Work out the finished part from the listing and answer in its coordinate system (mm). Give positions to 0.01 mm unless a question says otherwise; leave off trailing zeros. Write each loop counter-clockwise with the first axis right and the second up, starting at its lowest first coordinate (ties: lowest second). Pieces come first, ordered by that corner, then holes. Notation, with made-up numbers: (26.5, -9) - (52.5, -9) arc R25 ccw to (52.5, 12) - close; hole circle Ø4 at (87, 17). An arc over 180 degrees is marked (long way). Write item = value, one per line.
from build123d import *

# Parameters (mm, degrees)
F0_R     = 3.05
F0_R_2   = 2.5
F1_DEPTH = 5
F2_SIZE  = 3.5


with BuildPart() as f1:
    # F0 (on Top) → F1 (new body)
    with BuildSketch(Plane.XY):
        with BuildLine():
            Line((0, 225), (0, 0))
            Line((0, 0), (72.5, 0))
            ThreePointArc((72.5, 0), (86.642136, -5.857864), (92.5, -20))
            Line((92.5, -20), (92.5, -50))
            ThreePointArc((92.5, -50), (98.357864, -64.142136), (112.5, -70))
            Line((112.5, -70), (152.5, -70))
            ThreePointArc((152.5, -70), (166.642136, -64.142136), (172.5, -50))
            Line((172.5, -50), (172.5, -20))
            ThreePointArc((172.5, -20), (178.357864, -5.857864), (192.5, 0))
            Line((192.5, 0), (265, 0))
            Line((265, 0), (265, 225))
            Line((265, 225), (0, 225))
        make_face()
        with Locations((112.5, -50)):
            Circle(F0_R, mode=Mode.SUBTRACT)
        with Locations((112.5, -10)):
            Circle(F0_R, mode=Mode.SUBTRACT)
        with Locations((11, 35)):
            Circle(F0_R_2, mode=Mode.SUBTRACT)
        with Locations((11, 54.5)):
            Circle(F0_R_2, mode=Mode.SUBTRACT)
        with Locations((152.5, -50)):
            Circle(F0_R, mode=Mode.SUBTRACT)
        with Locations((152.5, -10)):
            Circle(F0_R, mode=Mode.SUBTRACT)
        with Locations((254, 35)):
            Circle(F0_R_2, mode=Mode.SUBTRACT)
        with Locations((254, 54.5)):
            Circle(F0_R_2, mode=Mode.SUBTRACT)
        with Locations((11, 170.5)):
            Circle(F0_R_2, mode=Mode.SUBTRACT)
        with Locations((11, 190)):
            Circle(F0_R_2, mode=Mode.SUBTRACT)
        with Locations((254, 170.5)):
            Circle(F0_R_2, mode=Mode.SUBTRACT)
        with Locations((254, 190)):
            Circle(F0_R_2, mode=Mode.SUBTRACT)
    extrude(amount=F1_DEPTH)

    # F2
    f2_edges = [f1.edges().sort_by_distance(p)[0] for p in [
        (109.45, -10, 5),
        (149.45, -10, 5),
        (109.45, -50, 5),
        (149.45, -50, 5),
    ]]
    chamfer(f2_edges, length=F2_SIZE)


solid = f1.part
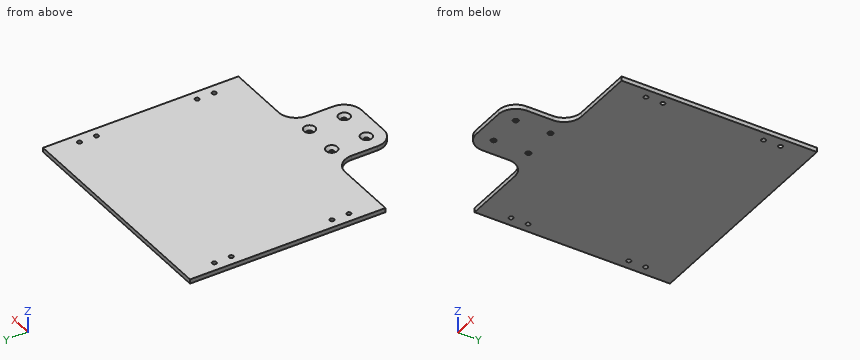
1. Find section B-B, the plane y = -33. Give the vertices of the cut face in (x, z), then the cut area to 3 significant figures.
Solution:
outline = (92.5, 0) - (172.5, 0) - (172.5, 5) - (92.5, 5) - close
area = 400 mm^2
2. Find section A-A, the plane z = 2.35. Give the number of separate pieces and of enclosed holes in the cut face, then the cut area to 3 significant figures.
Solution:
separate_pieces = 1
enclosed_holes = 12
area = 64,900 mm^2
3. Find section C-C, the plane x = 237.5. Give the vertices of the cut face in (y, z).
Solution:
outline = (0, 0) - (225, 0) - (225, 5) - (0, 5) - close
4. Straight lines are drawn through the part: line 1 (X direction, y = 190, z = 2.65); line 2 (Y direction, x = 11, z = 2.6); line 3 (Y direction, x = 112.5, z = 0.95). For each, find the intervals that lie inside material, in ascending order.
Solution:
line_1 = 0 to 8.5, 13.5 to 251.5, 256.5 to 265
line_2 = 0 to 32.5, 37.5 to 52, 57 to 168, 173 to 187.5, 192.5 to 225
line_3 = -70 to -53.05, -46.95 to -13.05, -6.95 to 225
5. Given pin 1 (2 mm diameter, centred on x = 201.5, z = 3, fed in from -Y); pin 2 (6 mm diameter, centred on x = 254, y = 35, fed in from -Z); pin 3 (7 mm diameter, centred on x = 112.5, y = -50, fed in from +Z); pin 4 (2.5 mm diameter, centred on y = -35, z = 3.5, fed in from -X), each flat-ended and moving along its own axis, determine where each tip first touches the part or whether it passes through.
Solution:
pin_1 = 0
pin_2 = 0
pin_3 = 1.95
pin_4 = 92.5
